from build123d import *

# Parameters (mm, degrees)
SKETCH2_R           = 15.278874537
BOSS_EXTRUDE1_DEPTH = 30
BOSS_EXTRUDE2_DEPTH = 30
CIRPATTERN1_COUNT   = 16


with BuildPart() as part:
    # Sketch2 → Boss-Extrude1 (new body)
    with BuildSketch(Plane.XY):
        Circle(SKETCH2_R)
    extrude(amount=BOSS_EXTRUDE1_DEPTH)

    # Sketch3 → Boss-Extrude2 (add)
    with BuildSketch(Plane(origin=(0, 0, 0), x_dir=(-1, 0, 0), z_dir=(0, 0, -1))):
        with BuildLine():
            Line((-2.735176163, 15.032059688), (-0.235176163, 17.532059688))
            Line((-0.235176163, 17.532059688), (0.235176163, 17.532059688))
            Line((0.235176163, 17.532059688), (2.735176163, 15.032059688))
            ThreePointArc((2.735176163, 15.032059688), (0, 15.278874537), (-2.735176163, 15.032059688))
        make_face()
    boss_extrude2 = extrude(amount=-BOSS_EXTRUDE2_DEPTH)

    # CirPattern1: Boss-Extrude2 ×16 about axis
    cirpattern1_axis = Axis((0, 0, 0), (0, 0, 1))
    for i in range(1, CIRPATTERN1_COUNT):
        add(boss_extrude2.rotate(cirpattern1_axis, i * 360 / CIRPATTERN1_COUNT))


solid = part.part
CAD build for the part. Positions are in the model's coordinates, mm. A direction names the side the tool comes from. Coordinates: 2 decimals unless noted, no trailing zeros. Write each loop counter-clockwise with the first axis right and the second up, starting at its lowest first coordinate (ties: lowest second). Pieces come first, ordered by that corner, then holes. Notation, with made-up numbers: (-2, 45) - (40, 45) arc R23 cw to (40, 68) - close; hole circle Ø7 at (77.5, 22.5). An arc over 180 degrees is marked (long way). Use a Markdown table: item, result. Add a question column.
Item 1: Mould opens along Y. For faces 1 (the face through (-16.3, -1.47, 14.79)), 2 (the face through (16.3, 1.47, 14.79)), 3 (the face through (0, 0, 30)), 4 (the face through (-1.47, 16.3, 14.79)) say: pulls with the +Y half, pulls with the -Y half, needs draft (parallel to the pull), parting line crosses it, or undercut.
Item 2: Drill centre lines: L1, parallel to Y at x = -15.5, z = 1.5; L2, parallel to X at y = 16, z = 11.75; L3, parallel to Y at x = 11.5, z = 11. Where is each one in solid material? Low to high. Write a range as from..to.
Item 3: Flat gauge pins, fed straight in: pin 1 (3 mm diameter, centred on y = 2.5, z = 5, fed in from +X); pin 2 (1.1 mm diameter, centred on y = -10, z = 16, fed in from +X); pin 3 (2 mm diameter, centred on y = 8, z = 9.5, fed in from +X). Where does each tip first touch, or does it go through?
Item 4: Band-saw the part on A-A, the plane x = -11. Give the cut face in (y, z), and give its area (3 significant figures).
Item 5: 3-axis set-ups, long thin cutter, end or side, ignore diameter. For faces 5 (the face through (12.563, -10, 15)), 6 (the face through (-1.503, -16.265, 14.79)), 7 (the face through (4.88, 15.62, 14.79)): which of +Z, -Z, +X, -X, +Y, -Y reach the whole face in a straight line?
Numbers:
| question | item | result |
|---|---|---|
| 1 | face 1 | undercut |
| 1 | face 2 | undercut |
| 1 | face 3 | needs draft |
| 1 | face 4 | pulls with the +Y half |
| 2 | L1 | -7.18..-4.59, -2.27..2.27, 4.59..7.18 |
| 2 | L2 | -6.97..-5.8, -1.77..1.77, 5.8..6.97 |
| 2 | L3 | -12.56..12.56 |
| 3 | pin 1 | x = 16.77 |
| 3 | pin 2 | x = 12.56 |
| 3 | pin 3 | x = 15.93 |
| 4 | outline | (-12.56, 0) - (12.56, 0) - (12.56, 30) - (-12.56, 30) - close |
| 4 | area | 754 mm2 |
| 5 | face 5 | +Z, -Z, +X, -Y |
| 5 | face 6 | +Z, -Z, -Y |
| 5 | face 7 | +Z, -Z, +Y |
